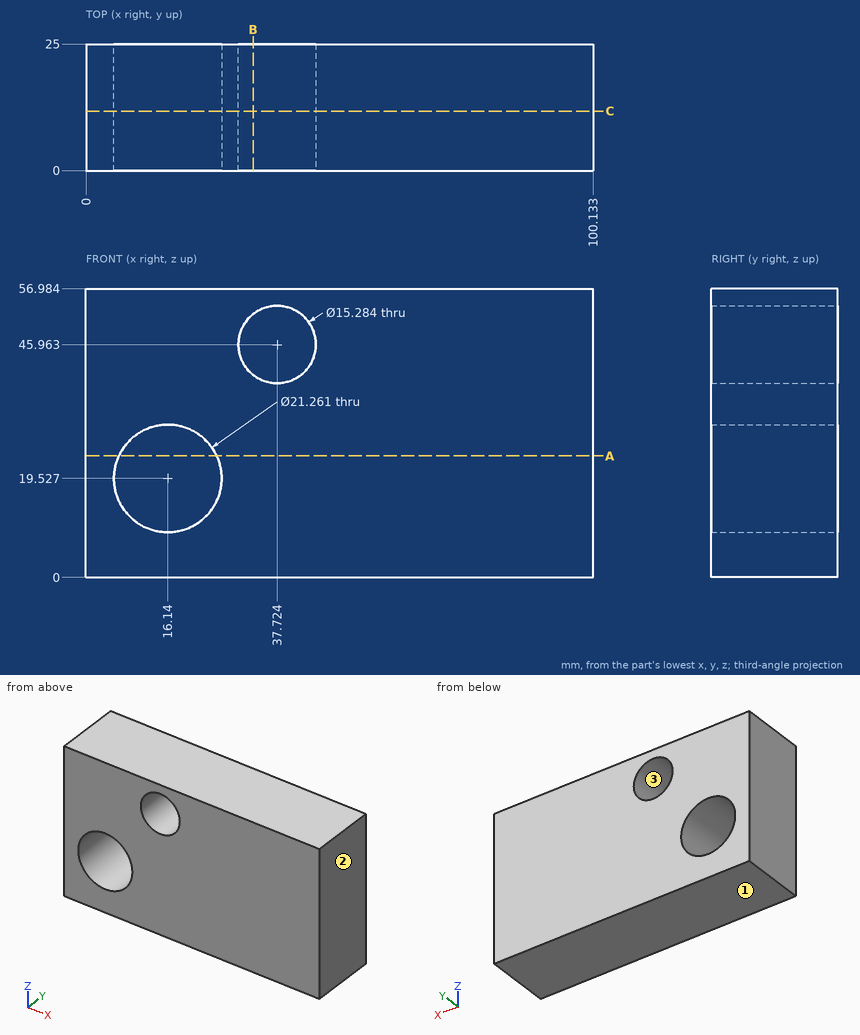
Geometry check sheet. Reference: drawing and pictorial views, mm from the part's lowest x, y, z. Give positions to 0.01 mm unless a question says otherwise; leave off trailing zeros. Order: outer loops, then holes, each group sorted by start corner. A loop starts at its lowest first (then second) coordinate and runs counter-clockwise, first axis right, second up. Notation, with made-up numbers: M 12,29.25 L 70,29.25 A18 cw 70,64.25 Z; hole C -1.5,53.25 d9. An arc over 180 degrees is marked long. Use one line per item in the form item = value. Start each with the question number.
Q1. Scan lines: line 1 along X through (y, z) = (21.5, 45) (1 decimal); line 2 along X through (y, z) = (8, 26) (1 decimal); line 3 along Z through (x, y) = (33, 20.5) (1 decimal). Record each from-to range of solid material in increasing order. Write a range as [from, to].
Q2. Section check B-B (x = 33). Enter the section's corners in (y, z) (1 decimal).
Q3. Mould release check, pull along Z, two halves, no side actions. Record for the marked faces 1, 2 and 3: +Z half, -Z half, draft (parallel to the pull), parting line (faces both ways), or undercut.
Q4. Section check C-C (y = 11.75). Enter the section's corners in (x, z) (1 decimal), then the cut area to 3 significant figures.
Q5. Section check A-A (z = 24). Enter the section's corners in (x, y) (1 decimal).
Evaluation:
q1.line_1 = [0, 30.1], [45.3, 100.1]
q1.line_2 = [0, 7.7], [24.6, 100.1]
q1.line_3 = [0, 40], [52, 57]
q2.outline = M 0,0 L 25,0 L 25,40 L 0,40 Z; M 0,52 L 25,52 L 25,57 L 0,57 Z
q3.face_1 = -Z half
q3.face_2 = draft
q3.face_3 = undercut
q4.outline = M 0,0 L 100.1,0 L 100.1,57 L 0,57 Z; hole C 16.1,19.5 d21.3; hole C 37.7,46 d15.3
q4.area = 5,170 mm2
q5.outline = M 0,0 L 6.5,0 L 6.5,25 L 0,25 Z; M 25.8,0 L 100.1,0 L 100.1,25 L 25.8,25 Z
